Part model, mm, in its own coordinate system. Give positions to 0.01 mm unless a question says otherwise; leave off trailing zeros. Write each loop counter-clockwise with the first axis right and the second up, starting at its lowest first coordinate (ties: lowest second). Pieces come first, ordered by that corner, then holes. Notation, with made-up numbers: M 69,2 L 101,2 A28 cw 101,34 Z; hole C 8,15 d2. An arc over 180 degrees is marked long. Write item = value, one per line. Start each with the question number.
from build123d import *

# Parameters (mm, degrees)
SZKIC1_R                    = 3
DODANIE_WYCI_GNI_CIE1_DEPTH = 2


with BuildPart() as part:
    # Szkic1 → Dodanie-wyciągnięcie1 (new body)
    with BuildSketch(Plane.XZ.offset(334.439810961)):
        with BuildLine():
            ThreePointArc((1003.4, 432.296579888), (1004.524695077, 431.895362049), (1005, 430.799916934))
            Line((1005, 430.799916934), (1015.903797979, 419.896118954))
            add(Edge.make_bspline(
                [(1015.903797979, 419.896118954), (1021.185746723, 422.066519939), (1027.589044834, 424.271723988), (1035, 426.42724062)],
                knots=[0.141934854, 0.141934854, 0.141934854, 0.141934854, 0.193423322, 0.193423322, 0.193423322, 0.193423322], degree=3, weights=[0.593424606, 0.563749359, 0.541143612, 0.525607364]))
            Line((1035, 426.42724062), (1035, 430.799916934))
            ThreePointArc((1035, 430.799916934), (1035.475304923, 431.895362049), (1036.6, 432.296579888))
            ThreePointArc((1036.6, 432.296579888), (1041.13903563, 442.62700703), (1031.039616452, 437.59488008))
            ThreePointArc((1031.039616452, 437.59488008), (1030.440005619, 435.425099056), (1028.5, 434.283231707))
            Line((1028.5, 434.283231707), (1011.5, 434.283231707))
            ThreePointArc((1011.5, 434.283231707), (1009.559994381, 435.425099056), (1008.960383548, 437.59488008))
            ThreePointArc((1008.960383548, 437.59488008), (998.86096437, 442.62700703), (1003.4, 432.296579888))
        make_face()
        with Locations((1003, 438.283231707)):
            Circle(SZKIC1_R, mode=Mode.SUBTRACT)
        with Locations((1037, 438.283231707)):
            Circle(SZKIC1_R, mode=Mode.SUBTRACT)
    extrude(amount=DODANIE_WYCI_GNI_CIE1_DEPTH)


solid = part.part
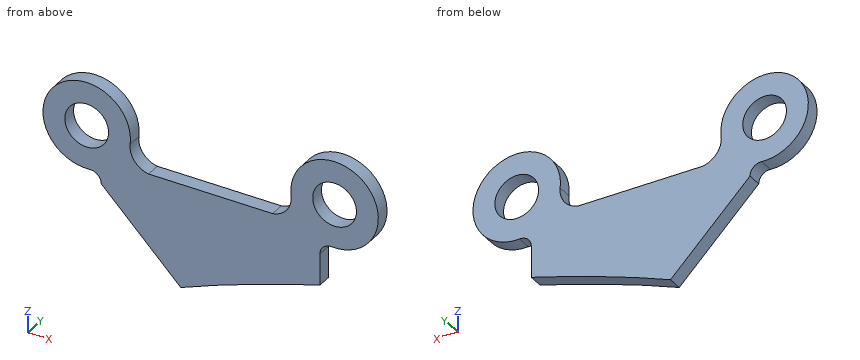
Q1. Probe line 1 along Z through (x, y) = (1003, -334.95); line 2 along X through (y, z) = (-335.25, 435.75); line 3 along X through (y, z) = (-336.1, 441). List the from-to ranges inside material, lowest first.
Q2. Drop flat-ended pins along their axis: P1, Ø5, axis at x = 1003, z = 438.28, coming from the +Y side; P2, Ø1, axis at y = -335, z = 427.5, coming from the +X side. Give the stop position or say it passes through.
Q3. Slice it at A-A (z = 437). Give the cut face in (x, y), and give its area (3 significant figures).
Q4. Slice it at D-D (z = 433.25). Give the cut face in (x, y).
Q5. Slice it at B-B (x = 1005.5). Give the cut face in (y, z).
Q6. Slice it at C-C (y = -336). Give the number of separate pieces and of enclosed holes in the cut face, and give its area (3 significant figures).
Working result:
q1.line_1 = 432.28 to 435.28, 441.28 to 444.28
q1.line_2 = 997.56 to 1001.39, 1004.61 to 1009.34, 1030.66 to 1035.39, 1038.61 to 1042.44
q1.line_3 = 997.65 to 1001.73, 1004.27 to 1008.35, 1031.65 to 1035.73, 1038.27 to 1042.35
q2.P1 = through
q2.P2 = 1035
q3.outline = M 997.14,-336.44 L 1000.29,-336.44 L 1000.29,-334.44 L 997.14,-334.44 Z; M 1005.71,-336.44 L 1008.95,-336.44 L 1008.95,-334.44 L 1005.71,-334.44 Z; M 1031.05,-336.44 L 1034.29,-336.44 L 1034.29,-334.44 L 1031.05,-334.44 Z; M 1039.71,-336.44 L 1042.86,-336.44 L 1042.86,-334.44 L 1039.71,-334.44 Z
q3.area = 25.6 mm2
q4.outline = M 999.73,-336.44 L 1040.27,-336.44 L 1040.27,-334.44 L 999.73,-334.44 Z
q5.outline = M -336.44,430.3 L -334.44,430.3 L -334.44,436.62 L -336.44,436.62 Z; M -336.44,439.94 L -334.44,439.94 L -334.44,443.74 L -336.44,443.74 Z
q6.separate_pieces = 1
q6.enclosed_holes = 2
q6.area = 480 mm2
